Check sheet for the modelled part. Datum: model origin and axes. Units: mm. A direction names the side the tool comes from. Give positions to 0.01 mm unless a question says otherwise; leave off trailing zeros. Loops run counter-clockwise (first coordinate to the right, second up) from the corner with the lowest first, then second, coordinate; pieces in that order, holes last. Notation, with made-up numbers: (49.5, 85.5) -> (57.5, 85.5) arc R26 cw to (57.5, 110.5) -> close; hole circle Ø9 at (-16.75, 22). An arc over 180 degrees is marked (long way). Answer as CSV lines item,"result". Start each with the question number.
(1) Material ranges on line 1 (Z direction, x = 0, y = 12.25); line 2 (Y direction, x = 0.5, z = 16); line 3 (Y direction, x = 11.5, z = 0), recorded low to high. Write a range as from..to.
(2) Section check B-B on z = -11.5. Enter the section's corners in (x, y), plus the area to 3 significant figures.
(3) Section check A-A on y = 76.5. Enter the section's corners in (x, z), plus the area to 3 significant figures.
(4) Gauge pin test, flat ends, axial feed: pin 1 Ø1.3 at (y, z) = (2.5, 0.5) entering from -X; pin 2 Ø3 at (y, z) = (44, -1) entering from +X; pin 3 Ø4.5 at (x, z) = (0, 0) entering from -Y; pin 4 Ø1 at (x, y) = (-13, 116.5) entering from +Z. Record the tip position at first contact, or that the pin passes through.
(5) Release check for a two-part mould opening along Y. For faces 5 (the face through (8, 8.7, -1.3)), 6 (the face through (0, 160, 0)), 7 (the face through (-10.648, -2.465, 13.887)), 8 (the face through (11, 10, 3)) record: pulls with the +Y half, pulls with the -Y half, needs draft (parallel to the pull), parting line crosses it, or undercut.
(6) Access from +Z, -Z, +X, -X, +Y, -Y to the whole of each face (thin tool, end or side, straight path). Record for faces 1 (the face through (4.708, 8.536, 0.325)), 2 (the face through (15, 81, 0)), 3 (the face through (-14.99, 78.88, -0.59)), 4 (the face through (1.5, 15, 0)).
from build123d import *

# Parameters (mm, degrees)
SKETCH1_R           = 15
BOSS_EXTRUDE1_DEPTH = 160
SKETCH2_W           = 0.857864376
SKETCH2_H           = 10
BOSS_EXTRUDE2_DEPTH = 160
SKETCH6_R           = 17.5
BOSS_EXTRUDE4_DEPTH = 5
CUT_EXTRUDE1_DEPTH  = 25
SKETCH4_R           = 1.5
CUT_EXTRUDE2_DEPTH  = 15
CUT_EXTRUDE3_REACH  = 171.903
CUT_EXTRUDE3_START  = 8
SKETCH7_R           = 3


with BuildPart() as part:
    # Sketch1 → Boss-Extrude1 (new body)
    with BuildSketch(Plane(origin=(0, 0, 0), x_dir=(1, 0, 0), z_dir=(0, 1, 0))):
        with Locations(Location((0, 0, 0), (0, 0, 270))):
            Circle(SKETCH1_R)
    extrude(amount=BOSS_EXTRUDE1_DEPTH)

    # Sketch2 → Boss-Extrude2 (add)
    with BuildSketch(Plane(origin=(0, 160, 0), x_dir=(1, 0, 0), z_dir=(0, 1, 0))):
        with Locations((14.571067812, 0)):
            Rectangle(SKETCH2_W, SKETCH2_H)
    extrude(amount=-BOSS_EXTRUDE2_DEPTH)

    # Sketch6 → Boss-Extrude4 (add)
    with BuildSketch(Plane.XZ):
        with Locations(Location((0, 0, 0), (0, 0, 270))):
            Circle(SKETCH6_R)
    extrude(amount=BOSS_EXTRUDE4_DEPTH)

    # Sketch3 → Cut-Extrude1 (cut)
    with BuildSketch(Plane.XZ.offset(5)):
        with BuildLine():
            Line((1.5, -1.322875656), (1.5, 1.322875656))
            ThreePointArc((1.5, 1.322875656), (-2, 0), (1.5, -1.322875656))
        make_face()
    extrude(amount=-CUT_EXTRUDE1_DEPTH, mode=Mode.SUBTRACT)

    # Sketch4 → Cut-Extrude2 (cut)
    with BuildSketch(Plane(origin=(15, 0, 0), x_dir=(0, 0, -1), z_dir=(1, 0, 0))):
        with Locations((0, 10)):
            Circle(SKETCH4_R)
    extrude(amount=-CUT_EXTRUDE2_DEPTH, mode=Mode.SUBTRACT)

    # Sketch7 → Cut-Extrude3 (cut, up to next)
    with BuildSketch(Plane(origin=(0, 0, 0), x_dir=(0, 0, -1), z_dir=(1, 0, 0)).offset(CUT_EXTRUDE3_START), mode=Mode.PRIVATE) as cut_extrude3_sk1:
        with Locations((0, 10)):
            Circle(SKETCH7_R)
    cut_extrude3_tool1 = extrude(cut_extrude3_sk1.sketch, amount=CUT_EXTRUDE3_REACH, mode=Mode.PRIVATE) & part.part
    add(cut_extrude3_tool1.solids().sort_by_distance((8, 10, 0))[0], mode=Mode.SUBTRACT)


solid = part.part
Working result:
1,line 1,"z = -15..-2, 2..15"
1,line 2,"y = -5..0"
1,line 3,"y = -5..7, 13..160"
2,outline,"(-13.19, -5) -> (13.19, -5) -> (13.19, 0) -> (9.63, 0) -> (9.63, 160) -> (-9.63, 160) -> (-9.63, 0) -> (-13.19, 0) -> close"
2,area,"3,210 mm^2"
3,outline,"(14.14, -5) -> (15, -5) -> (15, 5) -> (14.14, 5) arc R15 ccw (long way) to start"
3,area,"710 mm^2"
4,pin 1,"stops at x = -15"
4,pin 2,"stops at x = 15"
4,pin 3,"stops at y = -5"
4,pin 4,"stops at z = 8.29"
5,face 5,"undercut"
5,face 6,"pulls with the +Y half"
5,face 7,"needs draft"
5,face 8,"undercut"
6,face 1,"+X"
6,face 2,"+Z, -Z, +X, +Y"
6,face 3,"+Y"
6,face 4,"-Y"
